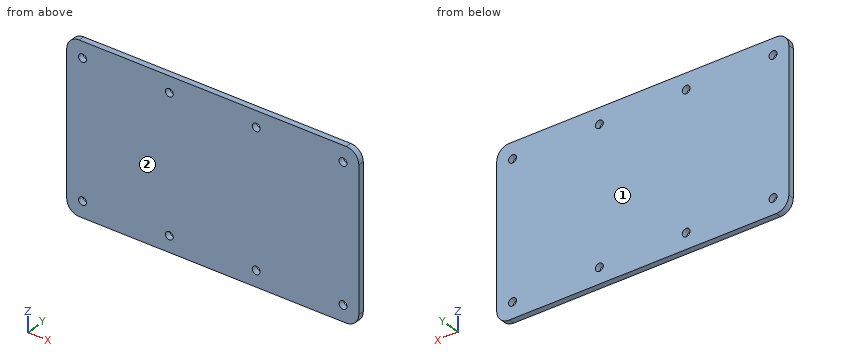
```python
from build123d import *

# Parameters (mm, degrees)
SKETCH1_W                   = 234.95
SKETCH1_H                   = 133.35
BOSS_EXTRUDE1_DEPTH         = 4.7625
FILLET1_R                   = 10.16
F_1_4_0_25_DIAMETER_HOLE3_D = 6.35


with BuildPart() as part:
    # Sketch1 → Boss-Extrude1 (new body)
    with BuildSketch(Plane(origin=(0, 0, 0), x_dir=(1, 0, 0), z_dir=(0, 1, 0))):
        with Locations((117.475, 66.675)):
            Rectangle(SKETCH1_W, SKETCH1_H)
    extrude(amount=BOSS_EXTRUDE1_DEPTH)

    # Fillet1
    fillet1_edges = [part.edges().sort_by_distance(p)[0] for p in [
        (0, 2.38125, -133.35),
        (234.95, 2.38125, -133.35),
        (234.95, 2.38125, 0),
        (0, 2.38125, 0),
    ]]
    fillet(fillet1_edges, radius=FILLET1_R)

    # 1/4 (0.25) Diameter Hole3 (through all)
    with Locations(Plane(origin=(0, 4.7625, 0), x_dir=(1, 0, 0), z_dir=(0, 1, 0))):
        with Locations((12.7, 120.65), (82.55, 120.65), (152.4, 120.65), (222.25, 120.65)):
            f_1_4_0_25_diameter_hole3 = Hole(F_1_4_0_25_DIAMETER_HOLE3_D / 2)

    # Mirror1: 1/4 (0.25) Diameter Hole3 across plane
    add(f_1_4_0_25_diameter_hole3.mirror(Plane.XY.offset(-66.675)), mode=Mode.SUBTRACT)


solid = part.part
```
For this review, take the finished solid that the model builds, in its own axes (mm). Face numbers are marked on the shaded views. Round coordinates to 2 decimals unless told otherwise and drop trailing zeros. Use one line per item in the form item = value.
Q1. To check wall thickness, follow probe 1 along Z at (x, y) = (12.7, 1.55) (3 decimals); probe 2 along X at (y, z) = (2.4, -120.65) (3 decimals); probe 3 along Z at (x, y) = (150, 0.2). State the ranges of each line that lie inside material, in increasing order. Write a range as from..to.
Resolved:
probe_1 = -133.35..-123.825, -117.475..-15.875, -9.525..0
probe_2 = 0..9.525, 15.875..79.375, 85.725..149.225, 155.575..219.075, 225.425..234.95
probe_3 = -133.35..-122.73, -118.57..-14.78, -10.62..0
Q2. The part is to be moulded in two halves that separate along Y. For the marked faces 1 and 2, say which applies: released by +Y, released by -Y, zero draft, split by the parting line, or undercut.
Resolved:
face_1 = released by +Y
face_2 = released by -Y
Q3. Consider section A-A (z = -120.65). State how many separate pieces and enclosed holes the cut face has, then the cut area to 3 significant figures.
Resolved:
separate_pieces = 5
enclosed_holes = 0
area = 998 mm²
Q4. Clearance check with a flat-ended pin moving along its axis: pin 1 Ø5.5 at (x, z) = (222.25, -120.65) entering from -Y. State where the tip first meets the part, or that it passes through.
Resolved:
pin_1 = through
